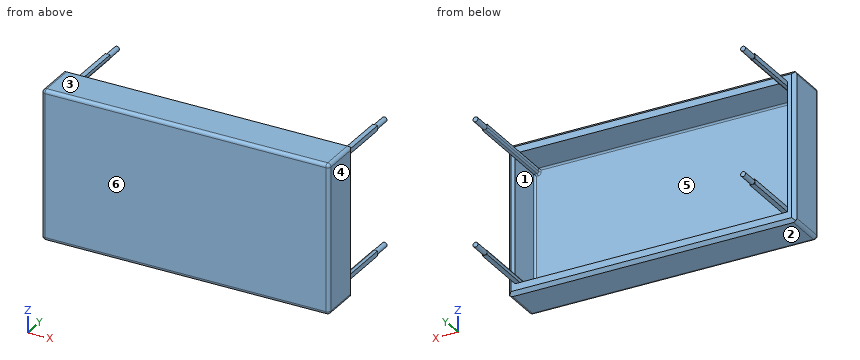
Autodesk Inventor part; units mm, degrees
ref_plane "YZ Plane" through (0, 0, 0) normal (1, 0, 0) x (0, 1, 0)
ref_plane "XZ Plane" through (0, 0, 0) normal (0, 1, 0) x (-1, 0, 0)
ref_plane "XY Plane" through (0, 0, 0) normal (0, 0, 1) x (1, 0, 0)
sketch "Sketch1" plane through (0, 0, 0) normal (0, 1, 0) x (-1, 0, 0)
  line L0 (-85.5, -44.5) -> (85.5, -44.5)
  line L1 (85.5, -44.5) -> (85.5, 44.5)
  line L2 (85.5, 44.5) -> (-85.5, 44.5)
  line L3 (-85.5, 44.5) -> (-85.5, -44.5)
  line L4 (-85.5, -44.5) -> (85.5, 44.5) construction
  line L5 (85.5, -44.5) -> (-85.5, 44.5) construction
  line L6 (-81, -38.5) -> (81, -38.5)
  line L7 (81, -38.5) -> (81, 38.5)
  line L8 (81, 38.5) -> (-81, 38.5)
  line L9 (-81, 38.5) -> (-81, -38.5)
  line L10 (-81, -38.5) -> (81, 38.5) construction
  line L11 (81, -38.5) -> (-81, 38.5) construction
  line L12 (81, 38.5) -> (79.55, 38.5)
  line L13 (81, 37.05) -> (81, 38.5)
  circle A0 centre (79.55, 37.05) radius 1.45
  circle A1 centre (79.55, -37.05) radius 1.45
  circle A2 centre (-79.55, -37.05) radius 1.45
  circle A3 centre (-79.55, 37.05) radius 1.45
  line L14 (81, 38.5) -> (78.1, 38.5)
  line L15 (78.1, 38.5) -> (78.1, 35.6)
  line L16 (78.1, 35.6) -> (81, 35.6)
  line L17 (81, 35.6) -> (81, 38.5)
  line L18 (81, 38.5) -> (78.1, 35.6) construction
  line L19 (78.1, 38.5) -> (81, 35.6) construction
  line L20 (81, -35.6) -> (78.1, -35.6)
  line L21 (78.1, -35.6) -> (78.1, -38.5)
  line L22 (78.1, -38.5) -> (81, -38.5)
  line L23 (81, -38.5) -> (81, -35.6)
  line L24 (81, -35.6) -> (78.1, -38.5) construction
  line L25 (78.1, -35.6) -> (81, -38.5) construction
  line L26 (-78.1, -35.6) -> (-81, -35.6)
  line L27 (-81, -35.6) -> (-81, -38.5)
  line L28 (-81, -38.5) -> (-78.1, -38.5)
  line L29 (-78.1, -38.5) -> (-78.1, -35.6)
  line L30 (-78.1, -35.6) -> (-81, -38.5) construction
  line L31 (-81, -35.6) -> (-78.1, -38.5) construction
  line L32 (-78.1, 38.5) -> (-81, 38.5)
  line L33 (-81, 38.5) -> (-81, 35.6)
  line L34 (-81, 35.6) -> (-78.1, 35.6)
  line L35 (-78.1, 35.6) -> (-78.1, 38.5)
  line L36 (-78.1, 38.5) -> (-81, 35.6) construction
  line L37 (-81, 38.5) -> (-78.1, 35.6) construction
  point P0 (0, 0)
  point P1 (-79.55, 38.5)
  point P2 (-81, 37.05)
  point P3 (-81, -37.05)
  point P4 (-79.55, -38.5)
  point P5 (79.55, -38.5)
  point P6 (81, -37.05)
  dimension "d0" = 171
  dimension "d1" = 89
  dimension "d2" = 162
  dimension "d3" = 77
  dimension "d7" = 2.9
  dimension "d8" = 2.9
  dimension "d9" = 2.9
  dimension "d10" = 2.9
extrude "Extrusion1" add sketch "Sketch1" along normal blind 70 contours A2 | A1 | A3 | A0
extrude "Extrusion2" add sketch "Sketch1" along normal blind 4 contours L29 L26 L9 L34 L35 L8 L15 L16 L7 L20 L21 L6 | L6 A2 L29 | L21 A1 L6 | A2 L26 L29 | L21 L20 A1 | L9 L26 A2 | A1 L20 L7 | L9 A3 L34 | L16 A0 L7 | A3 L35 L34 | L16 L15 A0 | L8 L35 A3 | A0 L15 L8
extrude "Extrusion3" add sketch "Sketch1" along normal blind 25
extrude "Extrusion4" add sketch "Sketch1" along normal blind 60 contours L6 L9 A2
extrude "Extrusion5" add sketch "Sketch1" along normal blind 60 contours L6 A2 L29 | L6 L9 A2 | A2 | A2 L26 L29 | L9 L26 A2
extrude "Extrusion6" add sketch "Sketch1" along normal blind 60 contours L9 A3 L34 | L9 L8 A3 | A3 | A3 L35 L34 | L8 L35 A3
extrude "Extrusion7" add sketch "Sketch1" along normal blind 60 contours L16 A0 L7 | A0 L8 L7 | A0 | L16 L15 A0 | A0 L15 L8
extrude "Extrusion8" add sketch "Sketch1" along normal blind 60 contours L21 A1 L6 | A1 L7 L6 | A1 | L21 L20 A1 | A1 L20 L7
fillet "Fillet1" radius 1 1 edges at (-78.1, 32, -35.6)
fillet "Fillet2" radius 1 1 edges at (-78.1, 32, 35.6)
fillet "Fillet3" radius 1 1 edges at (78.1, 32, 35.6)
fillet "Fillet4" radius 1 1 edges at (78.1, 32, -35.6)
fillet "Fillet5" radius 1 16 edges at (-81, 4, 0) (-78.1, 4, -37.55) (-80.05, 4, -35.6) (-78.3929, 4, -35.8929) (0, 4, -38.5) (0, 4, 38.5) (-78.3929, 4, 35.8929) (-80.05, 4, 35.6) (-78.1, 4, 37.55) (80.05, 4, -35.6) (78.1, 4, -37.55) (78.3929, 4, -35.8929) (81, 4, 0) (78.3929, 4, 35.8929) (80.05, 4, 35.6) (78.1, 4, 37.55)
chamfer "Chamfer1" distance 2 angle 45 4 edges at (0, 25, 44.5) (85.5, 25, 0) (0, 25, -44.5) (-85.5, 25, 0)
fillet "Fillet6" radius 2 1 edges at (85.5, 11.5, 44.5)
fillet "Fillet7" radius 2 1 edges at (85.5, 11.5, -44.5)
fillet "Fillet8" radius 2 1 edges at (-85.5, 11.5, 44.5)
fillet "Fillet9" radius 2 1 edges at (-85.5, 11.5, -44.5)
fillet "Fillet10" radius 2 4 edges at (-85.5, 0, 0) (0, 0, 44.5) (85.5, 0, 0) (0, 0, -44.5)
properties part number "Buggy_Body"
Design review of the part built by this model. Coordinates are the model's own, in mm. Face numbers are marked on the shaded views. A direction names the side the tool comes from. Round coordinates to 2 decimals unless told otherwise and drop trailing zeros. Write each loop counter-clockwise with the first axis right and the second up, starting at its lowest first coordinate (ties: lowest second). Pieces come first, ordered by that corner, then holes. Notation, with made-up numbers: (73.25, 46.5) -> (101.25, 46.5) arc R32 ccw to (101.25, 79.5) -> close; hole circle Ø1 at (21.25, -0.5). An arc over 180 degrees is marked (long way). Write item = value, one per line. Start each with the question number.
1) Take a section at C-C, the plane x = 48.5. State the section outline as (y, z) points, plus the area to 3 significant figures.
2) Tool access review of the marked faces 5 and 6: name each direction out of +Z, -Z, +X, -X, +Y, -Y from which nothing blocks a thin tool from reaching the whole face with its end or side.
3) Clearance check with flat-ended pins moving along their axes: pin 1 (1.5 mm diameter, centred on x = 79.5, y = 38, fed in from +Z); pin 2 (3 mm diameter, centred on x = 38.5, z = 31.5, fed in from +Y); pin 3 (1.5 mm diameter, centred on y = 24, z = -37, fed in from +X). State where each tip first meets the part, or that it passes through.
4) Take a section at A-A, the plane y = 54. State the section outline as (x, z) points.
5) Take a section at D-D, the plane y = 62. State the section outline as (x, z) points, plus the area to 3 significant figures.
6) Mouldability with a two-part tool opening along Z and no side actions: class the marked faces 1, 2, 3 and 4 as +Z half, -Z half, draft (parallel to the pull), parting line (faces both ways), or undercut.
7) Wall thickness on probe 1 along Z at (x, y) = (-19, 8.5); probe 2 along X at (y, z) = (15.5, 20.5); probe 3 along X at (y, z) = (47, -36.5): over which ranges is each line inside the solid? List them lowest first. Write a range as from..to.
8) Take a section at B-B, the plane z = -26.5. State the section outline as (x, y) points, plus the area to 3 significant figures.
Results list:
q1.outline = (0, -42.5) arc R2 ccw to (2, -44.5) -> (23, -44.5) -> (25, -42.5) -> (25, -38.5) -> (5, -38.5) arc R1 cw to (4, -37.5) -> (4, 37.5) arc R1 cw to (5, 38.5) -> (25, 38.5) -> (25, 42.5) -> (23, 44.5) -> (2, 44.5) arc R2 ccw to (0, 42.5) -> close
q1.area = 603 mm²
q2.face_5 = +Y
q2.face_6 = +Z, -Z, +X, -X, -Y
q3.pin_1 = 38.5
q3.pin_2 = 4
q3.pin_3 = 85.25
q4.outline = (-81, -38.5) -> (-78.1, -38.5) -> (-78.1, -36.6) arc R1 ccw to (-79.1, -35.6) -> (-81, -35.6) -> close; (-81, 35.6) -> (-79.1, 35.6) arc R1 ccw to (-78.1, 36.6) -> (-78.1, 38.5) -> (-81, 38.5) -> close; (78.1, -38.5) -> (81, -38.5) -> (81, -35.6) -> (79.1, -35.6) arc R1 ccw to (78.1, -36.6) -> close; (78.1, 36.6) arc R1 ccw to (79.1, 35.6) -> (81, 35.6) -> (81, 38.5) -> (78.1, 38.5) -> close
q5.outline = circle Ø2.9 at (-79.55, -37.05); circle Ø2.9 at (-79.55, 37.05); circle Ø2.9 at (79.55, -37.05); circle Ø2.9 at (79.55, 37.05)
q5.area = 26.4 mm²
q6.face_1 = undercut
q6.face_2 = -Z half
q6.face_3 = +Z half
q6.face_4 = draft
q7.probe_1 = -44.5..-38.5, 38.5..44.5
q7.probe_2 = -85.5..-81, 81..85.5
q7.probe_3 = -81..-78.11, 78.11..81
q8.outline = (-85.5, 2) arc R2 ccw to (-83.5, 0) -> (83.5, 0) arc R2 ccw to (85.5, 2) -> (85.5, 23) -> (83.5, 25) -> (81, 25) -> (81, 5) arc R1 cw to (80, 4) -> (-80, 4) arc R1 cw to (-81, 5) -> (-81, 25) -> (-83.5, 25) -> (-85.5, 23) -> close
q8.area = 868 mm²
